For this review, take the finished solid that the model builds, in its own axes (mm). A direction names the side the tool comes from. Coordinates: 2 decimals unless noted, no trailing zeros. Order: outer loops, then holes, each group sorted by start corner. A loop starts at its lowest first (then second) coordinate and runs counter-clockwise, first axis right, second up. Notation, with made-up numbers: (10, 87) -> (36, 87) arc R29 cw to (36, 113) -> close; hole circle Ø7 at (-23.5, 29.25). An arc over 180 degrees is marked (long way). Return JSON: item names as keys, results as strings. Group by question number.
Item 1: Take a section at A-A (x = -3.5). Write out the cut boundary in (y, z) (3 decimals), then the cut area to 3 significant figures.
Item 2: Draft analysis for pull direction Y (two halves, no side actions). For faces 1 (the cylindrical face through (23.02, 0.3, 0.76)), 2 (the cylindrical face through (-15.16, -19.43, -0.38)), 3 (the cylindrical face through (-23.02, -22.99, 8.3)), state which applies: +Y half, -Y half, draft (parallel to the pull), parting line (faces both ways), or undercut.
Item 3: Take a section at D-D (x = 18). Write out the cut boundary in (y, z), then the cut area to 3 significant figures.
Item 4: Take a section at C-C (z = 10.75). Count the separate pieces of the cut face and the enclosed holes in it, then the cut area to 3 significant figures.
Item 5: For line 1 along Y through (x, z) = (13, 7.75); line 2 along Y through (x, z) = (2, 11.5), list the stretches that pass through material, from the lowest coordinate up.
Item 6: Insertion check: pin 1 (1.7 mm diameter, centred on x = -15.81, y = -13.02, fed in from -Z); pin 2 (0.8 mm diameter, centred on y = -4.5, z = 2, fed in from +X); pin 3 (0.8 mm diameter, centred on y = -8, z = -0.5, fed in from -X). Each pin has a flat end and moves straight along its axis. Give the tip position at first contact, or say it passes through.
Item 7: Machinability: for faces 4 (the cylindrical face through (0.3, -23.02, 0.76)), 5 (the flat face through (0, 17.145, 1)), 6 (the flat face through (-16.129, -23, 12)), 7 (the flat face through (-18, 13, 0)), 8 (the flat face through (0, 22.479, 7)), which of the approach directions +Z, -Z, +X, -X, +Y, -Y give a long, thin tool a straight path to every point of the face, cutting with its end or side? Answer none if there is none.
Item 8: Take a section at B-B (z = 8.25). Write out the cut boundary in (x, y).
```python
from build123d import *

# Parameters (mm, degrees)
BOSS_EXTRUDE1_DEPTH     = 14.224
CUT_EXTRUDE1_DEPTH      = 11.684
FILLET1_R               = 2.54
SKETCH3_W               = 32.258
SKETCH3_H               = 8.128
CUT_EXTRUDE2_DEPTH      = 1
CUT_EXTRUDE2_DEPTH_BACK = 48.498
SKETCH5_W               = 26.924
SKETCH5_H               = 34.29
CUT_EXTRUDE4_DEPTH      = 1.524
SKETCH6_W               = 20.290608306
SKETCH6_H               = 27.072145664
CUT_EXTRUDE5_DEPTH      = 1.524
BOSS_EXTRUDE2_DEPTH     = 0.762
SKETCH8_W               = 12.7
SKETCH8_H               = 0.508
BOSS_EXTRUDE3_DEPTH     = 4.064


with BuildPart() as part:
    # Sketch1 → Boss-Extrude1 (new body)
    with BuildSketch(Plane.XY):
        with BuildLine():
            Line((-21.209, -23.749), (21.209, -23.749))
            ThreePointArc((21.209, -23.749), (23.005051224, -23.005051224), (23.749, -21.209))
            Line((23.749, -21.209), (23.749, 21.209))
            ThreePointArc((23.749, 21.209), (23.005051224, 23.005051224), (21.209, 23.749))
            Line((21.209, 23.749), (-21.209, 23.749))
            ThreePointArc((-21.209, 23.749), (-23.005051224, 23.005051224), (-23.749, 21.209))
            Line((-23.749, 21.209), (-23.749, -21.209))
            ThreePointArc((-23.749, -21.209), (-23.005051224, -23.005051224), (-21.209, -23.749))
        make_face()
    extrude(amount=BOSS_EXTRUDE1_DEPTH)

    # Sketch2 → Cut-Extrude1 (cut)
    with BuildSketch(Plane.XY.offset(14.224)):
        with BuildLine():
            Line((19.939, -22.479), (-19.939, -22.479))
            ThreePointArc((-19.939, -22.479), (-21.735051224, -21.735051224), (-22.479, -19.939))
            Line((-22.479, -19.939), (-22.479, 19.939))
            ThreePointArc((-22.479, 19.939), (-21.735051224, 21.735051224), (-19.939, 22.479))
            Line((-19.939, 22.479), (19.939, 22.479))
            ThreePointArc((19.939, 22.479), (21.735051224, 21.735051224), (22.479, 19.939))
            Line((22.479, 19.939), (22.479, -19.939))
            ThreePointArc((22.479, -19.939), (21.735051224, -21.735051224), (19.939, -22.479))
        make_face()
    extrude(amount=-CUT_EXTRUDE1_DEPTH, mode=Mode.SUBTRACT)

    # Fillet1
    fillet1_edges = [part.edges().sort_by_distance(p)[0] for p in [
        (0, -23.749, 0),
        (-23.005051224, -23.005051224, 0),
        (-23.749, 0, 0),
        (-23.005051224, 23.005051224, 0),
        (0, 23.749, 0),
        (23.005051224, 23.005051224, 0),
        (23.749, 0, 0),
        (23.005051224, -23.005051224, 0),
    ]]
    fillet(fillet1_edges, radius=FILLET1_R)

    # Sketch3 → Cut-Extrude2 (cut, two sides)
    with BuildSketch(Plane(origin=(0, 23.749, 0), x_dir=(1, 0, 0), z_dir=(0, 1, 0))) as cut_extrude2_sk:
        with Locations((0, -14.224)):
            Rectangle(SKETCH3_W, SKETCH3_H)
    extrude(amount=CUT_EXTRUDE2_DEPTH, mode=Mode.SUBTRACT)
    extrude(cut_extrude2_sk.sketch, amount=-CUT_EXTRUDE2_DEPTH_BACK, mode=Mode.SUBTRACT)

    # Sketch5 → Cut-Extrude4 (cut)
    with BuildSketch(Plane(origin=(0, 0, 0), x_dir=(-1, 0, 0), z_dir=(0, 0, -1))):
        Rectangle(SKETCH5_W, SKETCH5_H)
    extrude(amount=-CUT_EXTRUDE4_DEPTH, mode=Mode.SUBTRACT)

    # Sketch6 → Cut-Extrude5 (cut)
    with BuildSketch(Plane(origin=(0, 0, 1.524), x_dir=(-1, 0, 0), z_dir=(0, 0, -1))):
        Rectangle(SKETCH6_W, SKETCH6_H)
    extrude(amount=-CUT_EXTRUDE5_DEPTH, mode=Mode.SUBTRACT)

    # Sketch7 → Boss-Extrude2 (add)
    with BuildSketch(Plane(origin=(0, 0, 0), x_dir=(-1, 0, 0), z_dir=(0, 0, -1))):
        with BuildLine():
            Line((19.939, 17.145), (21.209, 17.145))
            ThreePointArc((21.209, 17.145), (17.399, 20.955), (13.589, 17.145))
            Line((13.589, 17.145), (14.859, 17.145))
            ThreePointArc((14.859, 17.145), (17.399, 19.685), (19.939, 17.145))
        make_face()
        with BuildLine():
            Line((21.209, 15.875), (16.129, 15.875))
            ThreePointArc((16.129, 15.875), (13.589, 13.335), (16.129, 10.795))
            Line((16.129, 10.795), (21.209, 10.795))
            Line((21.209, 10.795), (21.209, 12.065))
            Line((21.209, 12.065), (16.129, 12.065))
            ThreePointArc((16.129, 12.065), (14.859, 13.335), (16.129, 14.605))
            Line((16.129, 14.605), (21.209, 14.605))
            Line((21.209, 14.605), (21.209, 15.875))
        make_face()
        Polygon((13.589, 9.525), (21.209, 9.525), (21.209, 5.715), (19.939, 5.715), (19.939, 8.255), (18.034, 8.255), (18.034, 6.985), (16.764, 6.985), (16.764, 8.255), (13.589, 8.255), align=None)
        Polygon((13.589, 4.445), (21.209, 4.445), (21.209, 0.635), (19.939, 0.635), (19.939, 3.175), (18.034, 3.175), (18.034, 1.905), (16.764, 1.905), (16.764, 3.175), (13.589, 3.175), align=None)
        Polygon((21.209, -0.635), (13.589, -0.635), (13.589, -4.445), (14.859, -4.445), (14.859, -1.905), (21.209, -1.905), align=None)
        Polygon((13.589, -5.715), (21.209, -5.715), (21.209, -9.525), (19.939, -9.525), (19.939, -6.985), (18.034, -6.985), (18.034, -8.255), (16.764, -8.255), (16.764, -6.985), (14.859, -6.985), (14.859, -9.525), (13.589, -9.525), align=None)
        with BuildLine():
            Line((18.9865, -13.97), (18.9865, -15.24))
            ThreePointArc((18.9865, -15.24), (20.558044821, -11.445955179), (16.764, -13.0175))
            ThreePointArc((16.764, -13.0175), (15.137980791, -13.691019209), (15.8115, -12.065))
            Line((15.8115, -12.065), (15.8115, -10.795))
            ThreePointArc((15.8115, -10.795), (14.239955179, -14.589044821), (18.034, -13.0175))
            ThreePointArc((18.034, -13.0175), (19.660019209, -12.343980791), (18.9865, -13.97))
        make_face()
        with BuildLine():
            Line((15.8115, -17.78), (15.8115, -16.51))
            ThreePointArc((15.8115, -16.51), (14.239955179, -20.304044821), (18.034, -18.7325))
            ThreePointArc((18.034, -18.7325), (19.660019209, -18.058980791), (18.9865, -19.685))
            Line((18.9865, -19.685), (18.9865, -20.955))
            ThreePointArc((18.9865, -20.955), (20.558044821, -17.160955179), (16.764, -18.7325))
            ThreePointArc((16.764, -18.7325), (15.137980791, -19.406019209), (15.8115, -17.78))
        make_face()
    extrude(amount=BOSS_EXTRUDE2_DEPTH)

    # Sketch8 → Boss-Extrude3 (add)
    with BuildSketch(Plane.XY.offset(10.16)):
        with Locations((0, 22.733)):
            Rectangle(SKETCH8_W, SKETCH8_H)
        with Locations((0, -22.733)):
            Rectangle(SKETCH8_W, SKETCH8_H)
    extrude(amount=BOSS_EXTRUDE3_DEPTH)


solid = part.part
```
Findings below:
{
 "1": {"outline": "(-23.749, 2.54) arc R2.54 ccw to (-21.209, 0) -> (-17.145, 0) -> (-17.145, 1.524) -> (-13.536, 1.524) -> (-13.536, 2.54) -> (-22.479, 2.54) -> (-22.479, 14.224) -> (-22.987, 14.224) -> (-22.987, 10.16) -> (-23.749, 10.16) -> close; (13.536, 1.524) -> (17.145, 1.524) -> (17.145, 0) -> (21.209, 0) arc R2.54 ccw to (23.749, 2.54) -> (23.749, 10.16) -> (22.987, 10.16) -> (22.987, 14.224) -> (22.479, 14.224) -> (22.479, 2.54) -> (13.536, 2.54) -> close", "area": "61.6 mm2"},
 "2": {"face 1": "draft", "face 2": "undercut", "face 3": "-Y half"},
 "3": {"outline": "(-23.75, 2.54) arc R2.54 ccw to (-21.21, 0) -> (21.21, 0) arc R2.54 ccw to (23.75, 2.54) -> (23.75, 14.22) -> (22.48, 14.22) -> (22.48, 2.54) -> (-22.48, 2.54) -> (-22.48, 14.22) -> (-23.75, 14.22) -> close", "area": "148 mm2"},
 "4": {"separate pieces": "4", "enclosed holes": "0", "area": "166 mm2"},
 "5": {"line 1": "y = -23.75 to -22.48, 22.48 to 23.75", "line 2": "y = -22.99 to -22.48, 22.48 to 22.99"},
 "6": {"pin 1": "stops at z = 0", "pin 2": "stops at x = 23.75", "pin 3": "stops at x = -21.21"},
 "7": {"face 4": "-Z, +X, -X, -Y", "face 5": "-Z", "face 6": "+Z, +Y, -Y", "face 7": "-Z, -X", "face 8": "+Z"},
 "8": {"outline": "(-23.75, -21.21) arc R2.54 ccw to (-21.21, -23.75) -> (21.21, -23.75) arc R2.54 ccw to (23.75, -21.21) -> (23.75, 21.21) arc R2.54 ccw to (21.21, 23.75) -> (-21.21, 23.75) arc R2.54 ccw to (-23.75, 21.21) -> close; hole (-22.48, -19.94) arc R2.54 ccw to (-19.94, -22.48) -> (19.94, -22.48) arc R2.54 ccw to (22.48, -19.94) -> (22.48, 19.94) arc R2.54 ccw to (19.94, 22.48) -> (-19.94, 22.48) arc R2.54 ccw to (-22.48, 19.94) -> close"}
}
